Could you check a few things on this drawing? It's one solid part, dimensions in mm from its lowest x, y, z. Give positions to 0.01 mm unless a question says otherwise; leave off trailing zeros. Loops run counter-clockwise (first coordinate to the right, second up) from the corner with the lowest first, then second, coordinate; pieces in that order, holes last. Notation, with made-up numbers: (-12.5, 44) - (4.5, 44) arc R14 cw to (4.5, 63) - close; hole circle Ø5 at (-7, 54). An arc over 180 degrees is marked (long way). Use CSV: the item, a comma, the result in double quotes.
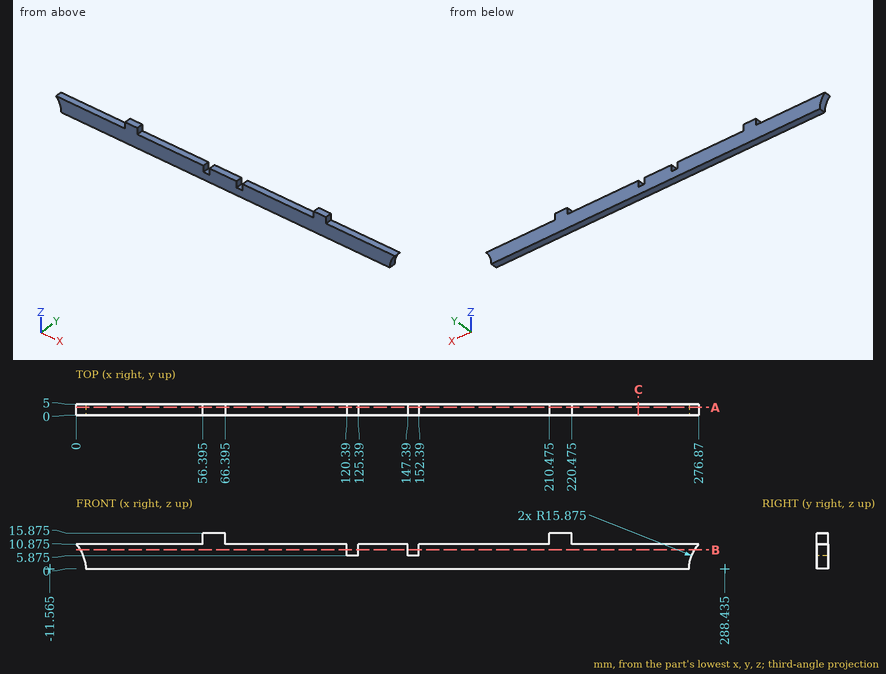
1) Suppose I cut it at C-C (x = 250). Please give me the cut outline in (y, z) (3 decimals), plus the area to 3 significant figures.
Answer below:
outline,"(0, 0) - (5, 0) - (5, 10.875) - (0, 10.875) - close"
area,"54.4 mm2"
2) Suppose I cut it at B-B (z = 8.5). Please give me the cut outline in (x, y).
Answer below:
outline,"(1.84, 0) - (120.39, 0) - (120.39, 5) - (1.84, 5) - close; (125.39, 0) - (147.39, 0) - (147.39, 5) - (125.39, 5) - close; (152.39, 0) - (275.03, 0) - (275.03, 5) - (152.39, 5) - close"
3) Suppose I cut it at A-A (y = 3.5). Please give me the cut outline in (x, z) (3 decimals), plus the area to 3 significant figures.
Answer below:
outline,"(0, 10.875) arc R15.875 cw to (4.31, 0) - (272.56, 0) arc R15.875 cw to (276.87, 10.875) - (220.475, 10.875) - (220.475, 15.875) - (210.475, 15.875) - (210.475, 10.875) - (152.39, 10.875) - (152.39, 5.875) - (147.39, 5.875) - (147.39, 10.875) - (125.39, 10.875) - (125.39, 5.875) - (120.39, 5.875) - (120.39, 10.875) - (66.395, 10.875) - (66.395, 15.875) - (56.395, 15.875) - (56.395, 10.875) - close"
area,"3,000 mm2"
4) I'm going to push flat-ended pins straight in: P1, Ø1.5, axis at x = 90.5, y = 1.5, coming from the +Z side (3 decimals); P2, Ø1.5, axis at y = 2.5, z = 14.5, coming from the +X side (3 decimals); P3, Ø1.5, axis at x = 123.5, y = 3, coming from the +Z side (3 decimals). Where does each tip first touch, or does it pass through?
Answer below:
P1,"stops at z = 10.875"
P2,"stops at x = 220.475"
P3,"stops at z = 5.875"
5) I need wall thicknesses on line 1 along X through (y, z) = (2.55, 13.5) (3 decimals); line 2 along X through (y, z) = (1.4, 7.75); line 3 along X through (y, z) = (3.8, 6). Which ranges of each line are inside material? Lowest first, please.
Answer below:
line 1,"x = 56.395 to 66.395, 210.475 to 220.475"
line 2,"x = 2.29 to 120.39, 125.39 to 147.39, 152.39 to 274.58"
line 3,"x = 3.13 to 120.39, 125.39 to 147.39, 152.39 to 273.74"
